Source: CAD feature listing. Evaluate the final solid. Frame: model axes, mm. Face numbers are marked on the shaded views. A direction names the side the tool comes from. Round coordinates to 2 decimals unless told otherwise and drop trailing zeros. Write each loop counter-clockwise with the first axis right and the second up, starting at its lowest first coordinate (ties: lowest second). Pieces come first, ordered by that corner, then holes. Notation, with made-up numbers: (-27, -18) -> (-2, -18) arc R22 ccw to (-2, -12) -> close; hole circle Ø11 at (28, 5). An arc over 180 degrees is marked (long way). Put each result on its own line as item: value.
```python
from build123d import *

# Parameters (mm, degrees)
SKETCH1_R               = 1.25
BOSS_EXTRUDE1_DEPTH     = 12
SKETCH2_R               = 1.75
BOSS_EXTRUDE2_DEPTH     = 1
FILLET1_R               = 0.5
CUT_EXTRUDE1_DEPTH      = 14.233480268
CUT_EXTRUDE1_DEPTH_BACK = 14.233480268
SKETCH3_R               = 0.4
CHAMFER1_SIZE           = 0.2


with BuildPart() as part:
    # Sketch1 → Boss-Extrude1 (new body)
    with BuildSketch(Plane(origin=(0, 0, 0), x_dir=(0, 0, -1), z_dir=(1, 0, 0))):
        Circle(SKETCH1_R)
    extrude(amount=BOSS_EXTRUDE1_DEPTH)

    # Sketch2 → Boss-Extrude2 (add)
    with BuildSketch(Plane(origin=(12, 0, 0), x_dir=(0, 0, -1), z_dir=(1, 0, 0))):
        Circle(SKETCH2_R)
    extrude(amount=BOSS_EXTRUDE2_DEPTH)

    # Fillet1
    fillet1_edges = [part.edges().sort_by_distance(p)[0] for p in [
        (12, 0, 1.25),
    ]]
    fillet(fillet1_edges, radius=FILLET1_R - 0.0001)  # a hair under: the kernel refuses the full size

    # Sketch3 → Cut-Extrude1 (cut, two sides: drawn at the far end of the back side and taken through both)
    with BuildSketch(Plane(origin=(0, 0, 0), x_dir=(1, 0, 0), z_dir=(0, 1, 0)).offset(-CUT_EXTRUDE1_DEPTH_BACK)):
        with Locations(Location((1.44, 0, 0), (0, 0, 270))):
            Circle(SKETCH3_R)
    extrude(amount=CUT_EXTRUDE1_DEPTH + CUT_EXTRUDE1_DEPTH_BACK, mode=Mode.SUBTRACT)

    # Chamfer1
    chamfer1_edges = [part.edges().sort_by_distance(p)[0] for p in [
        (0, 0, 1.25),
    ]]
    chamfer(chamfer1_edges, length=CHAMFER1_SIZE)


solid = part.part
```
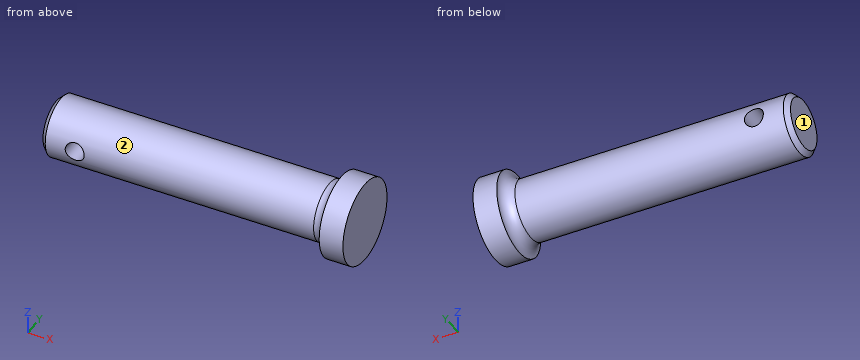
Q1. Cut plane D-D on x = 10. Output: boundary loops of the cut face in (y, z).
Ans:
outline: circle Ø2.5 at (0, 0)
Q2. Cut plane C-C on x = 1.44. Output: boundary loops of the cut face in (y, z), and give its area (3 significant figures).
Ans:
outline: (-1.18, -0.4) arc R1.25 ccw to (1.18, -0.4) -> close; (-1.18, 0.4) -> (1.18, 0.4) arc R1.25 ccw to start
area: 2.94 mm^2
Q3. Pin query (flat end, axial travel): pin 1 (1 mm diameter, centred on x = 3, y = -0.5, fed in from +Z); pin 2 (2 mm diameter, centred on x = 4, z = 0, fed in from +Y). Return the tip coordinate at first contact, or that it passes through.
Ans:
pin 1: stops at z = 1.25
pin 2: stops at y = 1.25
Q4. Material intervals for line 1 (X direction, y = 0.15, z = 0); line 2 (Z direction, x = 1.44, y = -0.6); line 3 (X direction, y = 0.15, z = 0.2), sorted ascending. Write a range as [from, to].
Ans:
line 1: x = [0, 1.04], [1.84, 13]
line 2: z = [-1.1, -0.4], [0.4, 1.1]
line 3: x = [0, 1.09], [1.79, 13]
Q5. Reachability of the marked faces 1 and 2 from +Z, -Z, +X, -X, +Y, -Y: full face, straight path, thin tool, end or side. Return the list, or none.
Ans:
face 1: +Z, -Z, -X, +Y, -Y
face 2: -X
